```python
from build123d import *

# Parameters (mm, degrees)
EXTRUDE_THIN1_DEPTH = 238.125
FILLET1_R           = 1.016


with BuildPart() as part:
    # Sketch1 → Extrude-Thin1 (new body)
    with BuildSketch(Plane.XY):
        with BuildLine():
            Line((0, 23.8125), (-15.875, 23.8125))
            Line((-15.875, 23.8125), (-15.875, 11.90625))
            Line((-15.875, 11.90625), (-13.49375, 11.90625))
            Line((-13.49375, 11.90625), (-13.49375, 9.525))
            ThreePointArc((-13.49375, 9.525), (-15.679243133, 8.08925057), (-15.229296459, 5.51334206))
            ThreePointArc((-15.229296459, 5.51334206), (-13.514036913, 2.963393123), (-12.7, 0))
            Line((-12.7, 0), (-10.31875, 0))
            Line((-10.31875, 0), (-10.31875, 1.016))
            Line((-10.31875, 1.016), (-11.826680113, 1.016))
            ThreePointArc((-11.826680113, 1.016), (-12.791218599, 3.800383088), (-14.488796637, 6.208982781))
            ThreePointArc((-14.488796637, 6.208982781), (-14.417167703, 8.149338041), (-12.47775, 8.05569932))
            Line((-12.47775, 8.05569932), (-12.47775, 12.92225))
            Line((-12.47775, 12.92225), (-14.859, 12.92225))
            Line((-14.859, 12.92225), (-14.859, 22.7965))
            Line((-14.859, 22.7965), (0, 22.7965))
            Line((0, 22.7965), (0, 23.8125))
        make_face()
    extrude(amount=-EXTRUDE_THIN1_DEPTH)

    # Fillet1
    fillet1_edges = [part.edges().sort_by_distance(p)[0] for p in [
        (-12.47775, 12.92225, -119.0625),
        (-12.47775, 8.05569932, -119.0625),
        (-12.7, 0, -119.0625),
        (-15.875, 11.90625, -119.0625),
        (-15.875, 23.8125, -119.0625),
    ]]
    fillet(fillet1_edges, radius=FILLET1_R)


solid = part.part
```
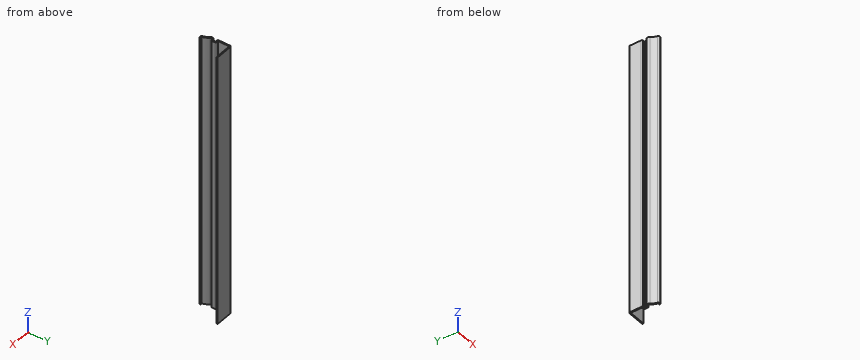
Design review of the part built by this model. Coordinates are the model's own, in mm. Give positions to 0.01 mm unless a question says otherwise; leave off trailing zeros. Order: outer loops, then holes, each group sorted by start corner. A loop starts at its lowest first (then second) coordinate and runs counter-clockwise, first axis right, second up. Notation, with made-up numbers: (-26, -3.5) - (30, -3.5) arc R22 cw to (30, 24.5) - close; hole circle Ø10 at (53.5, -20). An arc over 180 degrees is marked (long way). Use a Markdown table: item, result. Add a question column.
(1) Add section C-C on y = 3.5. Give the boundary of the cut face in (x, z) (3 decimals).
(2) Wall thickness on probe 1 along Y at (x, z) = (-10.75, -56); probe 2 along Y at (x, z) = (-7.75, -145); probe 3 along X at (y, z) = (21, -148.5) (3 decimals): over which ranges is each line inside the solid? List them lowest first. Write a range as [from, to].
(3) Clearance check with flat-ended pins moving along their axes: P1, Ø3, axis at x = -5.5, z = -117.5, coming from the -Y side; P2, Ø1.2, axis at y = 10.5, z = -111, coming from the -X side; P3, Ø1.2, axis at y = 10.5, z = -96.5, coming from the +X side. State where each tip first meets the part, or that it passes through.
(4) Add section B-B on x = -4.5. Give the boundary of the cut face in (y, z) (1 decimal).
Report:
| question | item | result |
|---|---|---|
| 1 | outline | (-13.781, -238.125) - (-12.643, -238.125) - (-12.643, 0) - (-13.781, 0) - close |
| 2 | probe 1 | y = [0, 1.02], [22.8, 23.81] |
| 2 | probe 2 | y = [22.8, 23.81] |
| 2 | probe 3 | x = [-15.875, -14.859] |
| 3 | P1 | stops at y = 22.8 |
| 3 | P2 | stops at x = -13.49 |
| 3 | P3 | stops at x = -12.48 |
| 4 | outline | (22.8, -238.1) - (23.8, -238.1) - (23.8, 0) - (22.8, 0) - close |
